from build123d import *

# Parameters (mm, degrees)
BOSS_EXTRUDE1_DEPTH = 2.8


with BuildPart() as part:
    # Sketch1 → Boss-Extrude1 (new body)
    with BuildSketch(Plane(origin=(0, 0, 0), x_dir=(1, 0, 0), z_dir=(0, 1, 0))):
        with BuildLine():
            Line((1.3, -17.4), (24.941531629, -17.4))
            ThreePointArc((24.941531629, -17.4), (27.53960784, -15.9), (27.53960784, -12.9))
            Line((27.53960784, -12.9), (15.718842026, 7.574166975))
            Line((15.718842026, 7.574166975), (9.310254038, 3.874166975))
            Line((9.310254038, 3.874166975), (8.010254038, 6.125833025))
            Line((8.010254038, 6.125833025), (14.418842026, 9.825833025))
            Line((14.418842026, 9.825833025), (2.598076211, 30.3))
            ThreePointArc((2.598076211, 30.3), (0, 31.8), (-2.598076211, 30.3))
            Line((-2.598076211, 30.3), (-14.418842026, 9.825833025))
            Line((-14.418842026, 9.825833025), (-8.010254038, 6.125833025))
            Line((-8.010254038, 6.125833025), (-9.310254038, 3.874166975))
            Line((-9.310254038, 3.874166975), (-15.718842026, 7.574166975))
            Line((-15.718842026, 7.574166975), (-27.53960784, -12.9))
            ThreePointArc((-27.53960784, -12.9), (-27.53960784, -15.9), (-24.941531629, -17.4))
            Line((-24.941531629, -17.4), (-1.3, -17.4))
            Line((-1.3, -17.4), (-1.3, -10))
            Line((-1.3, -10), (1.3, -10))
            Line((1.3, -10), (1.3, -17.4))
        make_face()
    extrude(amount=BOSS_EXTRUDE1_DEPTH)


solid = part.part
Input: part model. Units: mm. Frame: model coordinates. A direction names the side the tool comes from. Give positions to 0.01 mm unless a question says otherwise; leave off trailing zeros. Order: outer loops, then holes, each group sorted by start corner. A loop starts at its lowest first (then second) coordinate and runs counter-clockwise, first axis right, second up. Notation, with made-up numbers: (55.5, -18) - (94.5, -18) arc R12 cw to (94.5, 2) - close; hole circle Ø5 at (67.5, -19). An arc over 180 degrees is marked (long way). Answer as a JSON object with one key per item and string values. Group by question number.
Q1. Cut plane A-A, the plane y = 0.75. Output: boundary loops of the cut face in (x, z).
Q2. Set-up query: faces 5 (the face through (-11.26, 1.38, -8)), 6 (the face through (1.3, 1, 14)), 7 (the face through (0, 0, -2)). Return all of +Z, -Z, +X, -X, +Y, -Y with unobstructed straight access to the full face (end or side cutting, diameter ignored); none if empty.
Q3. Mould query, pull axis X, two halves, no side actions, for faces 1 (the face through (-8.65, 1.38, -5.02)), 2 (the face through (0, 1.4, -31.8)), 3 (the face through (8.59, 1.38, -19.92)), 4 (the face through (-8.426, 1.38, -20.206)). Classes: pulls with the +X half, pulls with the -X half, needs draft (parallel to the pull), parting line crosses it, or undercut.
Q4. First-contact query: pin 1 Ø1 at (y, z) = (2.5, -14) entering from +X; pin 2 Ø1.5 at (x, z) = (-3.5, -17.5) entering from -Y; pin 3 Ø1.3 at (x, y) = (0, 2) entering from +Z; pin 4 Ø0.8 at (y, z) = (1.5, 12.5) entering from -X. Flat tips, straight axial feed; report the tip coordinate or a pass-through.
Q5. Cut plane D-D, the plane x = 23.5. Output: boundary loops of the cut face in (y, z), then the cut area to 3 significant figures.
Q6. Cut plane C-C, the plane z = -14.5. Output: boundary loops of the cut face in (x, y), then the cut area to 3 significant figures.
Q7. Cut plane B-B, the plane x = -10. Output: boundary loops of the cut face in (y, z), then the cut area to 3 significant figures.
Q8. Line query: probe 1 along X at (y, z) = (0.7, -6.5); probe 2 along Z at (x, y) = (13, 0.4); probe 3 along X at (y, z) = (1.5, 11.5). Output: solid intervals per line, ascending.
Results:
{
 "1": {"outline": "(-27.54, 12.9) - (-15.72, -7.57) - (-9.31, -3.87) - (-8.01, -6.13) - (-14.42, -9.83) - (-2.6, -30.3) arc R3 ccw to (2.6, -30.3) - (14.42, -9.83) - (8.01, -6.13) - (9.31, -3.87) - (15.72, -7.57) - (27.54, 12.9) arc R3 ccw to (24.94, 17.4) - (1.3, 17.4) - (1.3, 10) - (-1.3, 10) - (-1.3, 17.4) - (-24.94, 17.4) arc R3 ccw to start"},
 "2": {"face 5": "+Y, -Y", "face 6": "+Z, +Y, -Y", "face 7": "+Z, -Z, +X, -X, -Y"},
 "3": {"face 1": "undercut", "face 2": "parting line crosses it", "face 3": "pulls with the +X half", "face 4": "pulls with the -X half"},
 "4": {"pin 1": "x = 12.3", "pin 2": "y = 0", "pin 3": "z = 10", "pin 4": "x = -27.54"},
 "5": {"outline": "(0, 5.9) - (2.8, 5.9) - (2.8, 17.4) - (0, 17.4) - close", "area": "32.2 mm^2"},
 "6": {"outline": "(-11.72, 0) - (11.72, 0) - (11.72, 2.8) - (-11.72, 2.8) - close", "area": "65.6 mm^2"},
 "7": {"outline": "(0, -17.48) - (2.8, -17.48) - (2.8, -7.27) - (0, -7.27) - close; (0, -4.27) - (2.8, -4.27) - (2.8, 17.4) - (0, 17.4) - close", "area": "89.3 mm^2"},
 "8": {"probe 1": "-16.34 to -13.86, -8.66 to 8.66, 13.86 to 16.34", "probe 2": "-12.28 to -9.01, -6 to 17.4", "probe 3": "-26.73 to -1.3, 1.3 to 26.73"}
}
